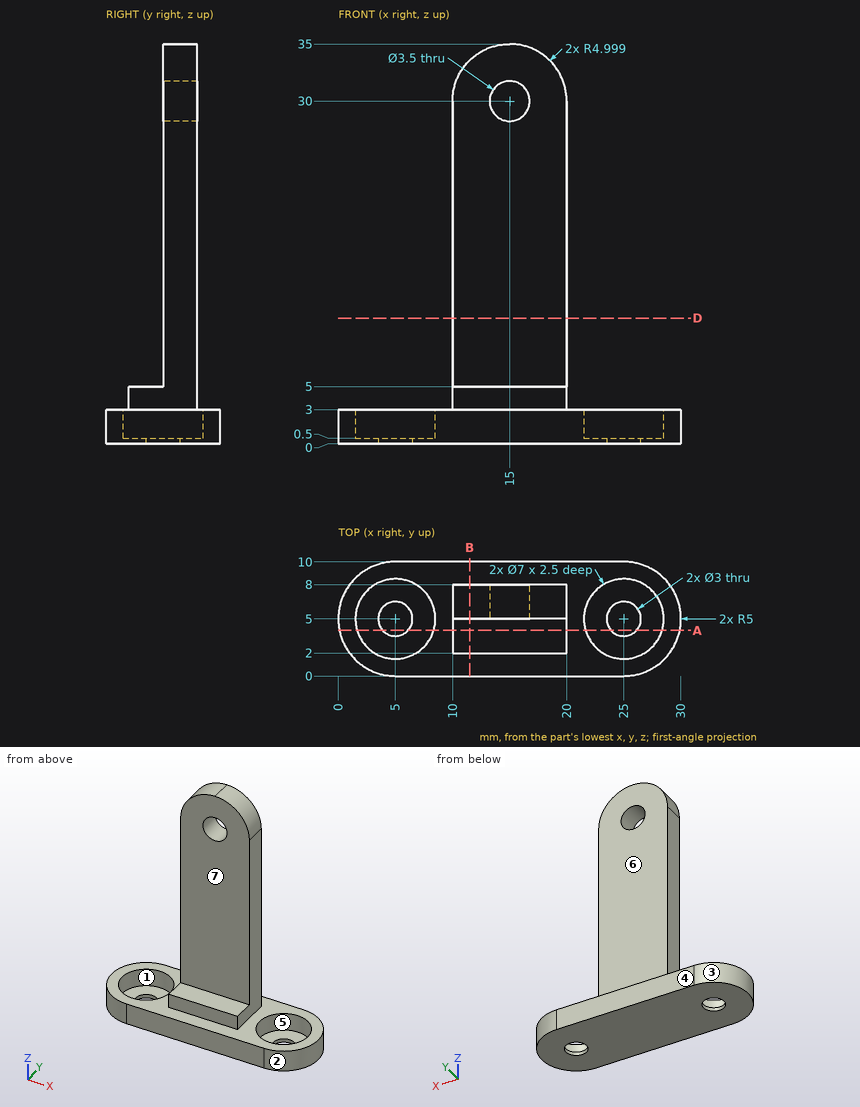
Answer from the drawing. Dimensions are ordinates in mm from the lowest x, y and z of the part. A direction names the side the tool comes from. Give positions to 0.01 mm unless a question says otherwise; leave off trailing zeros. Order: outer loops, then holes, each group sorted by start corner. A loop starts at its lowest first (then second) coordinate and runs counter-clockwise, first axis right, second up.
(1) For the marked faces 5, 6 and 7, determine the directions among +Z, -Z, +X, -X, +Y, -Y from which every point of the face is accessible in a straight line to the end or side of a thin tool.
(2) Find section D-D (z = 11). Give the vertices of the cut face in (x, y).
(3) Straight lines are drawn through the part: L1, parallel to X at y = 5, z = 0.35; L2, parallel to X at y = 5, z = 2.45; L3, parallel to Y at x = 5, z = 1.25. For each, find the intervals that lie inside material, in ascending order.
(4) Given pin 1 (3 mm diameter, centred on x = 18, z = 18, fed in from -Y); pin 2 (5.5 mm diameter, centred on x = 5, y = 6.5, fed in from +Z); pin 3 (1 mm diameter, centred on x = 14, z = 4.5, fed in from -Y); pin 4 (2 mm diameter, centred on x = 14.5, y = 6, fed in from +Z), each flat-ended and moving along its own axis, determine where each tip first touches the part or whether it passes through.
(5) Find section B-B (x = 11.5). Give the vertices of the cut face in (y, z), plus the area to 3 significant figures.
(6) Find section A-A (y = 4). Give the vertices of the cut face in (x, z).
(7) For a pull along X with two mould halves and no side action, classify the marked faces 1, 2, 3 and 4 as released by +X, released by -X, zero draft, split by the parting line, or undercut.
Result sheet:
1. face 5: +Z
1. face 6: +Z, +X, -X, +Y
1. face 7: +Z, +X, -X, -Y
2. outline: (10, 5) - (20, 5) - (20, 8) - (10, 8) - close
3. L1: x = 0 to 3.5, 6.5 to 23.5, 26.5 to 30
3. L2: x = 0 to 1.5, 8.5 to 21.5, 28.5 to 30
3. L3: y = 0 to 1.5, 8.5 to 10
4. pin 1: stops at y = 5
4. pin 2: stops at z = 3
4. pin 3: stops at y = 2
4. pin 4: stops at z = 35
5. outline: (0, 0) - (10, 0) - (10, 3) - (8, 3) - (8, 33.57) - (5, 33.57) - (5, 5) - (2, 5) - (2, 3) - (0, 3) - close
5. area: 128 mm2
6. outline: (0.1, 0) - (3.88, 0) - (3.88, 0.5) - (1.65, 0.5) - (1.65, 3) - (0.1, 3) - close; (6.12, 0) - (23.88, 0) - (23.88, 0.5) - (21.65, 0.5) - (21.65, 3) - (20, 3) - (20, 5) - (10, 5) - (10, 3) - (8.35, 3) - (8.35, 0.5) - (6.12, 0.5) - close; (26.12, 0) - (29.9, 0) - (29.9, 3) - (28.35, 3) - (28.35, 0.5) - (26.12, 0.5) - close
7. face 1: undercut
7. face 2: released by +X
7. face 3: released by -X
7. face 4: zero draft
